```python
from build123d import *

# Parameters (mm, degrees)
PAD6965_DEPTH            = 146.05
POCKET670_DEPTH          = 25.401
SKETCH7925_R             = 2.38125
POCKET674_DEPTH          = 25.401
BODY6271_PLACEMENT_ANGLE = 90


with BuildPart() as part:
    # Sketch7919 → Pad6965 (new body, symmetric)
    with BuildSketch(Plane.YZ):
        Polygon((0, 0), (0, -25.4), (3.175, -25.4), (3.175, -3.175), (25.4, -3.175), (25.4, 0), align=None)
    extrude(amount=PAD6965_DEPTH, both=True)

    # Sketch7920 → Pocket670 (cut, through all)
    with BuildSketch(Plane.XZ):
        Polygon((-107.95, -38.1), (-146.05, 0), (-146.05, -38.1), align=None)
        Polygon((107.95, -38.1), (146.05, 0), (146.05, -38.1), align=None)
    extrude(amount=-POCKET670_DEPTH, mode=Mode.SUBTRACT)

    # Sketch7925 → Pocket674 (cut, through all)
    with BuildSketch(Plane.XY):
        with Locations((-60.325, 12.7)):
            Circle(SKETCH7925_R)
        with Locations((60.325, 12.7)):
            Circle(SKETCH7925_R)
    extrude(amount=-POCKET674_DEPTH, mode=Mode.SUBTRACT)


with BuildPart() as part_1:
    # Body6271 placement: moved
    add(part.part.moved(Location((152.4, 0, -15.875))).rotate(Axis((152.4, 0, -15.875), (0, 1, 0)), BODY6271_PLACEMENT_ANGLE))


solid = part_1.part
```
Geometry: final body of the model. Coordinates: model frame, mm. A direction names the side the tool comes from. Round coordinates to 2 decimals unless told otherwise and drop trailing zeros. Loops run counter-clockwise (first coordinate to the right, second up) from the corner with the lowest first, then second, coordinate; pieces in that order, holes last. Notation, with made-up numbers: (6, -17.75) -> (54, -17.75) arc R20 cw to (54, -11.75) -> close; hole circle Ø3 at (-22, 15). An arc over 180 degrees is marked (long way). Use one line per item in the form item = value.
Item 1: Material intervals for probe 1 along Y at (x, z) = (151.05, 44.45); probe 2 along X at (y, z) = (24, -15.5) (3 decimals); probe 3 along Y at (x, z) = (146.5, 25) (3 decimals), sorted ascending.
Evaluation:
probe_1 = 0 to 10.32, 15.08 to 25.4
probe_2 = 149.225 to 152.4
probe_3 = 0 to 3.175
Item 2: Cut plane C-C on x = 138. Output: boundary loops of the cut face in (y, z) (3 decimals), then the cut area to 3 significant figures.
Evaluation:
outline = (0, -147.525) -> (3.175, -147.525) -> (3.175, 115.775) -> (0, 115.775) -> close
area = 836 mm2
Item 3: Cut plane A-A on y = 12.7. Output: boundary loops of the cut face in (x, z) (3 decimals).
Evaluation:
outline = (149.225, -158.75) -> (152.4, -161.925) -> (152.4, -78.581) -> (149.225, -78.581) -> close; (149.225, -73.819) -> (152.4, -73.819) -> (152.4, 42.069) -> (149.225, 42.069) -> close; (149.225, 46.831) -> (152.4, 46.831) -> (152.4, 130.175) -> (149.225, 127) -> close
Item 4: Contact query for flat-ended pins moving along their axis: pin 1 Ø1 at (y, z) = (13, -19.5) entering from -X (3 decimals); pin 2 Ø3 at (y, z) = (12.7, 44.45) entering from -X; pin 3 Ø11 at (x, z) = (137.5, 21) entering from +Y (3 decimals); pin 4 Ø12 at (x, y) = (136, 8.5) entering from -Z. Output: stop coordinate, or through.
Evaluation:
pin_1 = 149.225
pin_2 = through
pin_3 = 3.175
pin_4 = -148.29
Item 5: Draft query along Y for faces 1 (the flat face through (144.344, 2.293, 122.119)), 2 (the flat face through (138, 3.175, -18)), 3 (the cylindrical face through (150.83, 12.8, 46.83)). Return one class per face: released by +Y, released by -Y, zero draft, split by the parting line, or undercut.
Evaluation:
face_1 = zero draft
face_2 = released by +Y
face_3 = undercut
Item 6: Cut plane B-B on z = 44.45. Output: boundary loops of the cut face in (x, y) (3 decimals).
Evaluation:
outline = (127, 0) -> (152.4, 0) -> (152.4, 10.319) -> (149.225, 10.319) -> (149.225, 3.175) -> (127, 3.175) -> close; (149.225, 15.081) -> (152.4, 15.081) -> (152.4, 25.4) -> (149.225, 25.4) -> close
Item 7: Access query for faces 4 (the flat face through (149.225, 14, -18)), 5 (the flat face through (140, 0, -18)). Directions: +Z, -Z, +X, -X, +Y, -Y. A direction counts if a zero-diameter tool reaches every point of the face in a straight line with its end or side. Return the directions, or none.
Evaluation:
face_4 = +Z, -Z, -X, +Y
face_5 = +Z, -Z, +X, -X, -Y
